Input: part model. Units: mm. Frame: model coordinates. Face numbers are marked on the shaded views. A direction names the side the tool comes from. Coordinates: 2 decimals unless noted, no trailing zeros. Write each loop counter-clockwise with the first axis right and the second up, starting at its lowest first coordinate (ties: lowest second). Pieces come first, ordered by that corner, then holes. Notation, with made-up numbers: M -20.5,21.5 L 11.5,21.5 A15 ccw 11.5,39.5 Z; hole C 78,41.25 d6. An arc over 180 degrees is marked long. Answer as a JSON object with one key per item and string values. Group by question number.
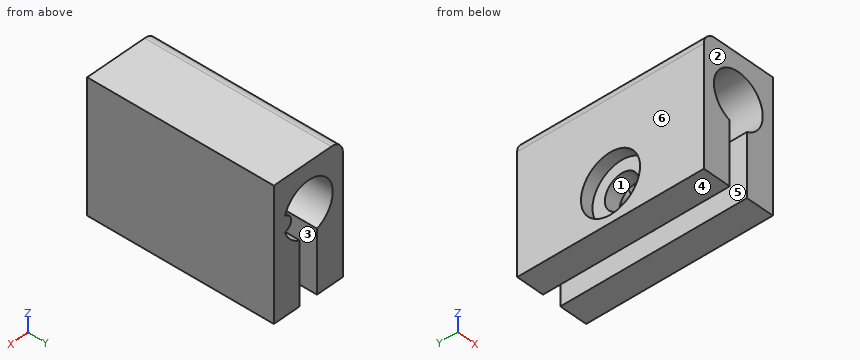
Autodesk Inventor part; units mm, degrees
ref_plane "YZ Plane" through (0, 0, 0) normal (1, 0, 0) x (0, 1, 0)
ref_plane "XZ Plane" through (0, 0, 0) normal (0, 1, 0) x (-1, 0, 0)
ref_plane "XY Plane" through (0, 0, 0) normal (0, 0, 1) x (1, 0, 0)
sketch "Sketch1" plane through (0, 0, 0) normal (0, 1, 0) x (-1, 0, 0)
  circle A0 centre (0, 0) radius 4.25
  line L0 (6, 7) -> (-6, 7)
  line L1 (-6, 7) -> (-6, -7)
  line L2 (-6, -7) -> (6, -7)
  line L3 (6, -7) -> (6, 7)
  line L4 (6, 7) -> (-6, 7)
  line L5 (-6, 7) -> (-6, 14)
  line L6 (-6, 14) -> (6, 14)
  line L7 (6, 14) -> (6, 7)
  point P0 (-6, 7)
  dimension "d0" = 8.5
  dimension "d1" = 6
  dimension "d2" = 14
  dimension "d3" = 12
  dimension "d4" = 7
  dimension "d5" = 7
extrude "Extrusion1" add sketch "Sketch1" along normal blind 35
sketch "Sketch2" plane through (0, 35, 0) normal (0, 1, 0) x (1, 0, 0)
  line L0 (-1.5, -16.1218) -> (1.5, -16.1218)
  line L1 (1.5, -16.1218) -> (1.5, -1.7668)
  line L2 (1.5, -1.7668) -> (-1.5, -1.7668)
  line L3 (-1.5, -1.7668) -> (-1.5, -16.1218)
  point P0 (0, 0)
  dimension "d8" = 1.5
  dimension "d9" = 1.5
extrude "Extrusion2" cut sketch "Sketch2" against normal through all
sketch "Sketch3" plane through (-6, 0, -7) normal (-1, 0, 0) x (0, 0, 1)
  circle A0 centre (15, 15) radius 2.75
  line L0 (21, 0) -> (21, 35)
  line L1 (0, 0) -> (21, 0)
  point P0 (7, 0)
  dimension "d12" = 5.5
  dimension "d13" = 6
  dimension "d14" = 15
extrude "Extrusion3" cut sketch "Sketch3" against normal blind 10
sketch "Sketch4" plane through (0, 35, 0) normal (0, 1, 0) x (1, 0, 0)
  arc A0 (1.5, -3.9765) -> (-1.5, -3.9765) centre (0, 0) ccw
  circle A1 centre (4.25, 0) radius 1.25
  point P0 (4.0662, 1.2364)
  point P1 (4.0662, -1.2364)
  dimension "d17" = 2.5
extrude "Extrusion4" add sketch "Sketch4" against normal blind 14.5 contours A1 A0 picked at (3.8196, 0)
sketch "Sketch5" plane through (0, 35, 0) normal (0, 1, 0) x (1, 0, 0)
  line L0 (1.5, -14) -> (6, -14)
  line L1 (6, -14) -> (36, -14)
  line L2 (36, -14) -> (36, 7)
  line L3 (36, 7) -> (6, 7)
  line L4 (6, 7) -> (6, -14)
  circle A0 centre (21, -3.5) radius 2.75
  point P0 (0, 0)
  dimension "d20" = 30
  dimension "d21" = 15
  dimension "d22" = 10.5
  dimension "d23" = 5.5
extrude "Extrusion5" add sketch "Sketch5" against normal blind 5
sketch "Sketch6" plane through (0, 35, 0) normal (0, 1, 0) x (1, 0, 0)
  circle A0 centre (21, -3.5) radius 2.75
  circle A1 centre (21, -3.5) radius 4.75
  point P0 (0, 0)
  dimension "d26" = 9.5
extrude "Extrusion6" cut sketch "Sketch6" against normal blind 2
sketch "Sketch7" plane through (-6, 0, -7) normal (-1, 0, 0) x (0, 0, 1)
  circle A0 centre (15, 15) radius 2.75
  circle A1 centre (15, 15) radius 4.75
  point P0 (7, 0)
  dimension "d29" = 9.5
extrude "Extrusion7" cut sketch "Sketch7" against normal blind 2
fillet "Fillet1" radius 2 3 edges at (-6, 17.5, -7) (36, 32.5, -7) (36, 32.5, 14)
sketch "Sketch9" plane through (0, 35, 0) normal (0, 1, 0) x (1, 0, 0)
  line L0 (-21.5057, -29.1514) -> (41.8439, -29.1514)
  line L1 (41.8439, -29.1514) -> (41.8439, 16.5719)
  line L2 (41.8439, 16.5719) -> (-21.5057, 16.5719)
  line L3 (-21.5057, 16.5719) -> (-21.5057, -29.1514)
  point P0 (0, 0)
extrude "Extrusion8" cut sketch "Sketch9" against normal blind 5
mirror "Mirror1" about plane through (6, 0, -7) normal (0, 0, -1) of "Extrusion1", "Extrusion2", "Extrusion3", "Extrusion4", "Extrusion5", "Extrusion6", "Extrusion7", "Fillet1", "Extrusion8"
sketch "Sketch10" plane through (-6, 0, -5) normal (-1, 0, 0) x (0, 0, 1)
  line L0 (-2, 30) -> (-2, 0)
  line L1 (26.294, -8.8637) -> (-2, -8.8637)
  line L2 (-2, -8.8637) -> (-2, 30)
  line L3 (-2, 30) -> (26.294, 30)
  line L4 (26.294, 30) -> (26.294, -8.8637)
  point P0 (5, 0)
  point P1 (-2, 0)
extrude "Extrusion9" cut sketch "Sketch10" against normal through all
properties part number "YsupportB"
Q1. Access query for the marked faces 1, 2 and 3. Directions: +Z, -Z, +X, -X, +Y, -Y. A direction counts if a zero-diameter tool reaches every point of the face in a straight line with its end or side. Return the directions, or none.
Q2. Section B-B, the plane z = -22. Return the cut outline in (x, y).
Q3. Draft query along X for the marked faces 4, 5 and 6. Return one class per face: released by +X, released by -X, zero draft, split by the parting line, or undercut.
Q4. Line query: line 1 (Y direction, x = -5.3, z = -22); line 2 (X direction, y = 17.25, z = -19); line 3 (Y direction, x = -2.05, z = -22). Output: solid intervals per line, ascending. Write a range as from..to.
Q5. Pin query (flat end, axial travel): pin 1 Ø3.5 at (y, z) = (15, -22) entering from -X. Return the tip coordinate at first contact, or that it passes through.
Q6. Section D-D, the plane y = 16.25. Return the cut outline in (x, z), and give its area (3 significant figures).
Q7. Section C-C, the plane z = -18.5. Return the cut outline in (x, y), and give its area (3 significant figures).
Q8. Section A-A, the plane x = -2. Return the cut outline in (y, z).
Filled in:
{
 "1": {"face 1": "-X", "face 2": "+Z, -Z, +X, -X, -Y", "face 3": "-Z, +Y, -Y"},
 "2": {"outline": "M -6,0 L -1.5,0 L -1.5,12.25 L -4,12.25 L -4,10.25 L -6,10.25 Z; M -6,19.75 L -4,19.75 L -4,17.75 L -1.5,17.75 L -1.5,30 L -6,30 Z; M 1.5,0 L 6,0 L 6,30 L 1.5,30 L 1.5,17.75 L 4,17.75 L 4,12.25 L 1.5,12.25 Z"},
 "3": {"face 4": "zero draft", "face 5": "undercut", "face 6": "released by -X"},
 "4": {"line 1": "0..10.25, 19.75..30", "line 2": "-4..-1.5, 1.5..6", "line 3": "0..12.25, 17.75..30"},
 "5": {"pin 1": "x = 4"},
 "6": {"outline": "M -6,-28 L -1.5,-28 L -1.5,-24.45 L -4,-24.45 L -4,-26.58 L -6,-26.58 Z; M -6,-17.42 L -4,-17.42 L -4,-19.55 L -1.5,-19.55 L -1.5,-17.98 A4.25 cw long 1.5,-17.98 L 1.5,-19.55 L 4,-19.55 L 4,-24.45 L 1.5,-24.45 L 1.5,-28 L 6,-28 L 6,-7 L -4,-7 A2 ccw -6,-9 Z", "area": "122 mm^2"},
 "7": {"outline": "M -6,0 L -1.5,0 L -1.5,30 L -6,30 L -6,18.21 L -4,18.21 L -4,11.79 L -6,11.79 Z; M 1.5,0 L 6,0 L 6,30 L 1.5,30 Z", "area": "257 mm^2"},
 "8": {"outline": "M 0,-28 L 30,-28 L 30,-17.75 L 0,-17.75 Z; M 0,-10.25 L 30,-10.25 L 30,-7 L 0,-7 Z; hole C 15,-22 d5.5"}
}
